The model under review builds one solid part; all positions refer to its coordinate system, in mm. A direction names the side the tool comes from. Give positions to 0.01 mm unless a question says otherwise; leave off trailing zeros. Order: outer loops, then holes, each group sorted by start corner. A loop starts at its lowest first (then second) coordinate and runs counter-clockwise, first axis right, second up. Notation, with made-up numbers: (76, -6) -> (127, -6) arc R9 ccw to (127, 9) -> close; hole circle Ø10 at (65.5, 33.25). An arc over 180 degrees is marked (long way). Answer as a JSON object with one key per item and string values. Group by question number.
from build123d import *

# Parameters (mm, degrees)
SKETCH3_W           = 100
SKETCH3_H           = 40
BOSS_EXTRUDE1_DEPTH = 19.05
SKETCH4_R           = 3
SKETCH4_R_2         = 6.35
CUT_EXTRUDE1_DEPTH  = 58.121821575
SKETCH5_R           = 6.35
CUT_EXTRUDE2_DEPTH  = 3


with BuildPart() as part:
    # Sketch3 → Boss-Extrude1 (new body)
    with BuildSketch(Plane(origin=(0, 0, 0), x_dir=(1, 0, 0), z_dir=(0, 1, 0))):
        Rectangle(SKETCH3_W, SKETCH3_H)
    extrude(amount=BOSS_EXTRUDE1_DEPTH)

    # Sketch4 → Cut-Extrude1 (cut, through all)
    with BuildSketch(Plane(origin=(0, 19.05, 0), x_dir=(1, 0, 0), z_dir=(0, 1, 0))):
        with Locations(Location((0, 9.55, 0), (0, 0, 270))):
            Circle(SKETCH4_R)
        with Locations(Location((0, -9.55, 0), (0, 0, 270))):
            Circle(SKETCH4_R)
        with Locations(Location((-30, 0, 0), (0, 0, 270))):
            Circle(SKETCH4_R_2)
        with Locations(Location((30, 0, 0), (0, 0, 270))):
            Circle(SKETCH4_R_2)
    extrude(amount=-CUT_EXTRUDE1_DEPTH, mode=Mode.SUBTRACT)

    # Sketch5 → Cut-Extrude2 (cut)
    with BuildSketch(Plane(origin=(0, 19.05, 0), x_dir=(1, 0, 0), z_dir=(0, 1, 0))):
        with Locations(Location((0, 9.55, 0), (0, 0, 270))):
            Circle(SKETCH5_R)
        with Locations(Location((0, -9.55, 0), (0, 0, 270))):
            Circle(SKETCH5_R)
    extrude(amount=-CUT_EXTRUDE2_DEPTH, mode=Mode.SUBTRACT)

    # Chamfer1
    # the kernel refuses this chamfer: 1, 0.363970234 mm, written as the material it takes off along each edge
    with BuildSketch(Plane(origin=(-49.757353177, 18.595343255, 19.333333333), x_dir=(0.34202014332567077, 0.9396926207859077, 0), z_dir=(-0.932495167133386, 0.3394004844336423, 0.12353167382937617))) as chamfer1_piece_1:
        Polygon((-0.595445134, 0.335906163), (0.468732639, 0.335906163), (0.126712495, -0.671812326), align=None)
    extrude(amount=0.509225374, mode=Mode.SUBTRACT)
    with BuildSketch(Plane(origin=(-49.545343255, 18.383333333, -19.757353177), x_dir=(-0.9396926207859077, 0, 0.34202014332567077), z_dir=(-0.3394004844336423, 0.12353167382937617, -0.932495167133386)), Plane(origin=(49.757353177, 18.595343255, 19.333333333), x_dir=(-0.34202014332567077, 0.9396926207859077, 0), z_dir=(0.932495167133386, 0.3394004844336423, 0.12353167382937617)), Plane(origin=(49.545343255, 0.242646823, -19.333333333), x_dir=(0.34202014332567077, 0, 0.9396926207859077), z_dir=(0.3394004844336414, -0.9324951671333863, -0.12353167382937585))) as chamfer1_piece_2:
        Polygon((-0.595445134, -0.335906163), (0.468732639, -0.335906163), (0.126712495, 0.671812326), align=None)
    extrude(amount=0.509225374, mode=Mode.SUBTRACT)
    with BuildSketch(Plane(origin=(-49.545343255, 0.242646823, 19.333333333), x_dir=(0.9396926207859081, -0.3420201433256699, 0), z_dir=(-0.3394004844336414, -0.9324951671333863, 0.12353167382937585))) as chamfer1_piece_3:
        Polygon((-0.468732639, -0.335906163), (0.595445134, -0.335906163), (-0.126712495, 0.671812326), align=None)
    extrude(amount=0.509225374, mode=Mode.SUBTRACT)
    with BuildSketch(Plane(origin=(49.757353177, 18.383333333, -19.545343255), x_dir=(0.34202014332567077, 0, 0.9396926207859077), z_dir=(0.932495167133386, 0.12353167382937617, -0.3394004844336423)), Plane(origin=(49.545343255, 0.242646823, 19.333333333), x_dir=(-0.9396926207859081, -0.3420201433256699, 0), z_dir=(0.3394004844336414, -0.9324951671333863, 0.12353167382937585)), Plane(origin=(-49.333333333, 0.242646823, -19.545343255), x_dir=(-0.9396926207859077, 0, 0.34202014332567077), z_dir=(-0.12353167382937585, -0.9324951671333863, -0.3394004844336414))) as chamfer1_piece_4:
        Polygon((-0.468732639, 0.335906163), (0.595445134, 0.335906163), (-0.126712495, -0.671812326), align=None)
    extrude(amount=0.509225374, mode=Mode.SUBTRACT)
    with BuildSketch(Plane(origin=(-50, 19.05, 22.594194733), x_dir=(-0.013184058198643421, -0.9999130865277317, 0), z_dir=(0, 0, -1)), Plane(origin=(50, 19.05, -22.594194733), x_dir=(0.013184058198643421, -0.9999130865277317, 0), z_dir=(0, 0, 1))) as chamfer1_piece_5:
        with BuildLine():
            Line((1.037677893, 0), (-0.042563411, -0.377122659))
            Line((-0.042563411, -0.377122659), (-0.062561673, -0.376858977))
            ThreePointArc((-0.062561673, -0.376858977), (-0.022487748, -0.188545427), (-0.019998262, 0.000263681))
            Line((-0.019998262, 0.000263681), (0.000263681, 0.019998262))
            ThreePointArc((0.000263681, 0.019998262), (0.519012443, 0.013158453), (1.037941574, 0.019998262))
            Line((1.037941574, 0.019998262), (1.037677893, 0))
        make_face()
    extrude(amount=45.188389465, mode=Mode.SUBTRACT)
    with BuildSketch(Plane(origin=(-50, -2.594194733, 20), x_dir=(-0.013184058198643421, 0, -0.9999130865277317), z_dir=(0, 1, 0)), Plane(origin=(-50, -2.594194733, -20), x_dir=(0.9999130865277315, 0, -0.013184058198646842), z_dir=(0, 1, 0))) as chamfer1_piece_6:
        with BuildLine():
            Line((1.037677893, 0), (-0.042563411, -0.377122659))
            Line((-0.042563411, -0.377122659), (-0.062561673, -0.376858977))
            ThreePointArc((-0.062561673, -0.376858977), (-0.022487748, -0.188545427), (-0.019998262, 0.000263681))
            Line((-0.019998262, 0.000263681), (0.000263681, 0.019998262))
            ThreePointArc((0.000263681, 0.019998262), (0.519012443, 0.013158453), (1.037941574, 0.019998262))
            Line((1.037941574, 0.019998262), (1.037677893, 0))
        make_face()
    extrude(amount=24.238389465, mode=Mode.SUBTRACT)
    with BuildSketch(Plane(origin=(52.594194733, 19.05, 20), x_dir=(0, 0.013184058198646846, -0.9999130865277317), z_dir=(-1, 0, 0))) as chamfer1_piece_7:
        with BuildLine():
            Line((1.037677893, 0), (-0.042563411, 0.377122659))
            Line((-0.042563411, 0.377122659), (-0.062561673, 0.376858977))
            ThreePointArc((-0.062561673, 0.376858977), (-0.022487748, 0.188545427), (-0.019998262, -0.000263681))
            Line((-0.019998262, -0.000263681), (0.000263681, -0.019998262))
            ThreePointArc((0.000263681, -0.019998262), (0.519012443, -0.013158453), (1.037941574, -0.019998262))
            Line((1.037941574, -0.019998262), (1.037677893, 0))
        make_face()
    extrude(amount=105.188389465, mode=Mode.SUBTRACT)
    with BuildSketch(Plane(origin=(50, -2.594194733, 20), x_dir=(0.013184058198643421, 0, -0.9999130865277317), z_dir=(0, 1, 0))) as chamfer1_piece_8:
        with BuildLine():
            Line((1.037677893, 0), (-0.042563411, 0.377122659))
            Line((-0.042563411, 0.377122659), (-0.062561673, 0.376858977))
            ThreePointArc((-0.062561673, 0.376858977), (-0.022487748, 0.188545427), (-0.019998262, -0.000263681))
            Line((-0.019998262, -0.000263681), (0.000263681, -0.019998262))
            ThreePointArc((0.000263681, -0.019998262), (0.519012443, -0.013158453), (1.037941574, -0.019998262))
            Line((1.037941574, -0.019998262), (1.037677893, 0))
        make_face()
    extrude(amount=24.238389465, mode=Mode.SUBTRACT)
    with BuildSketch(Plane(origin=(50, -2.594194733, -20), x_dir=(-0.9950833631817483, 0, -0.09904090225205378), z_dir=(0, 1, 0))) as chamfer1_piece_9:
        with BuildLine():
            Line((0.379516987, 0), (-0.116377165, 1.031131304))
            Line((-0.116377165, 1.031131304), (-0.136278832, 1.029150486))
            ThreePointArc((-0.136278832, 1.029150486), (-0.071283478, 0.514262313), (-0.019901667, -0.001980818))
            Line((-0.019901667, -0.001980818), (0.001980818, -0.019901667))
            ThreePointArc((0.001980818, -0.019901667), (0.189877952, -0.001200217), (0.381497805, -0.019901667))
            Line((0.381497805, -0.019901667), (0.379516987, 0))
        make_face()
    extrude(amount=24.238389465, mode=Mode.SUBTRACT)
    with BuildSketch(Plane(origin=(52.594194733, 0, 20), x_dir=(0, -0.013184058198645909, -0.9999130865277317), z_dir=(-1, 0, 0)), Plane(origin=(-52.594194733, 19.05, -20), x_dir=(0, -0.9999130865277315, -0.013184058198646842), z_dir=(1, 0, 0))) as chamfer1_piece_10:
        with BuildLine():
            Line((1.037677893, 0), (-0.042563411, -0.377122659))
            Line((-0.042563411, -0.377122659), (-0.062561673, -0.376858977))
            ThreePointArc((-0.062561673, -0.376858977), (-0.022487748, -0.188545427), (-0.019998262, 0.000263681))
            Line((-0.019998262, 0.000263681), (0.000263681, 0.019998262))
            ThreePointArc((0.000263681, 0.019998262), (0.519012443, 0.013158453), (1.037941574, 0.019998262))
            Line((1.037941574, 0.019998262), (1.037677893, 0))
        make_face()
    extrude(amount=105.188389465, mode=Mode.SUBTRACT)
    with BuildSketch(Plane(origin=(-50, 0, 22.594194733), x_dir=(-0.0990409022520534, 0.9950833631817484, 0), z_dir=(0, 0, -1)), Plane(origin=(50, 0, -22.594194733), x_dir=(0.0990409022520534, 0.9950833631817484, 0), z_dir=(0, 0, 1))) as chamfer1_piece_11:
        with BuildLine():
            Line((0.379516987, 0), (-0.116377165, 1.031131304))
            Line((-0.116377165, 1.031131304), (-0.136278832, 1.029150486))
            ThreePointArc((-0.136278832, 1.029150486), (-0.071283478, 0.514262313), (-0.019901667, -0.001980818))
            Line((-0.019901667, -0.001980818), (0.001980818, -0.019901667))
            ThreePointArc((0.001980818, -0.019901667), (0.189877952, -0.001200217), (0.381497805, -0.019901667))
            Line((0.381497805, -0.019901667), (0.379516987, 0))
        make_face()
    extrude(amount=45.188389465, mode=Mode.SUBTRACT)
    with BuildSketch(Plane(origin=(-52.594194733, 0, -20), x_dir=(0, 0.9950833631817482, -0.09904090225205339), z_dir=(1, 0, 0))) as chamfer1_piece_12:
        with BuildLine():
            Line((0.379516987, 0), (-0.116377165, 1.031131304))
            Line((-0.116377165, 1.031131304), (-0.136278832, 1.029150486))
            ThreePointArc((-0.136278832, 1.029150486), (-0.071283478, 0.514262313), (-0.019901667, -0.001980818))
            Line((-0.019901667, -0.001980818), (0.001980818, -0.019901667))
            ThreePointArc((0.001980818, -0.019901667), (0.189877952, -0.001200217), (0.381497805, -0.019901667))
            Line((0.381497805, -0.019901667), (0.379516987, 0))
        make_face()
    extrude(amount=105.188389465, mode=Mode.SUBTRACT)


solid = part.part
1. Take a section at D-D on x = -30. Give the boundary of the cut face in (y, z), plus the area to 3 significant figures.
2. Draft analysis for pull direction X (two halves, no side actions). For faces 1 (the flat face through (-1, 9, 20)), 2 (the flat face through (50, 9, 0)), 3 (the cylindrical face through (36.3, 9.7, -0.8)), 4 (the flat face through (-50, 9, 0)), state which applies: pulls with the +X half, pulls with the -X half, needs draft (parallel to the pull), parting line crosses it, or undercut.
3. For probe 1 along X at (y, z) = (9.5, 0); probe 2 along X at (y, z) = (7.5, 1.5); probe 3 along Z at (x, y) = (-2.5, 6), list the stretches that pass through material, from the lowest coordinate up. Write a range as [from, to].
4. For pin 1 (11.5 mm diameter, centred on x = -30, z = 0, fed in from -Y); pin 2 (7.5 mm diameter, centred on x = 0, z = 9.55, fed in from +Y), all flat-tipped, find the tip position at first contact; note any pin that passes through.
5. Take a section at C-C on z = 9.55. Give the boundary of the cut face in (x, y).
6. Take a section at A-A on z = 0. Give the boundary of the cut face in (x, y), plus the area to 3 significant figures.
7. Machinability: for faces 5 (the cylindrical face through (-28.093, 9.658, 6.057)), 6 (the cylindrical face through (-3.86, 17.57, 4.51)), which of the approach directions +Z, -Z, +X, -X, +Y, -Y give a long, thin tool a straight path to every point of the face, cutting with its end or side? Answer none if there is none.
8. Take a section at B-B on y = 1.5. Give the boundary of the cut face in (x, z).
Checks:
{
 "1": {"outline": "(0, -19) -> (0.36, -20) -> (18.05, -20) -> (19.05, -19.64) -> (19.05, -6.35) -> (0, -6.35) -> close; (0, 6.35) -> (19.05, 6.35) -> (19.05, 19) -> (18.69, 20) -> (0.36, 20) -> (0, 19) -> close", "area": "519 mm2"},
 "2": {"face 1": "needs draft", "face 2": "pulls with the +X half", "face 3": "undercut", "face 4": "pulls with the -X half"},
 "3": {"probe 1": "x = [-50, -36.35], [-23.65, 23.65], [36.35, 50]", "probe 2": "x = [-50, -36.17], [-23.83, 23.83], [36.17, 50]", "probe 3": "z = [-20, -11.21], [-7.89, 7.89], [11.21, 20]"},
 "4": {"pin 1": "passes through", "pin 2": "stops at y = 16.05"},
 "5": {"outline": "(-50, 0.36) -> (-49, 0) -> (-3, 0) -> (-3, 16.05) -> (-6.35, 16.05) -> (-6.35, 19.05) -> (-49.64, 19.05) -> (-50, 18.05) -> close; (3, 0) -> (49, 0) -> (50, 0.36) -> (50, 18.05) -> (49.64, 19.05) -> (6.35, 19.05) -> (6.35, 16.05) -> (3, 16.05) -> close"},
 "6": {"outline": "(-50, 0.36) -> (-49, 0) -> (-36.35, 0) -> (-36.35, 19.05) -> (-49.64, 19.05) -> (-50, 18.05) -> close; (-23.65, 0) -> (23.65, 0) -> (23.65, 19.05) -> (-23.65, 19.05) -> close; (36.35, 0) -> (49, 0) -> (50, 0.36) -> (50, 18.05) -> (49.64, 19.05) -> (36.35, 19.05) -> close", "area": "1,420 mm2"},
 "7": {"face 5": "+Y, -Y", "face 6": "+Y"},
 "8": {"outline": "(-50, -19.64) -> (-49, -20) -> (49.64, -20) -> (50, -19) -> (50, 19) -> (49.64, 20) -> (-49.64, 20) -> (-50, 19) -> close; hole circle Ø12.7 at (-30, 0); hole circle Ø6 at (0, -9.55); hole circle Ø6 at (0, 9.55); hole circle Ø12.7 at (30, 0)"}
}
